Input: part model. Units: mm. Frame: model coordinates. Face numbers are marked on the shaded views. A direction names the side the tool comes from. Round coordinates to 2 decimals unless told otherwise and drop trailing zeros. Write each loop counter-clockwise with the first axis right and the second up, starting at its lowest first coordinate (ties: lowest second). Pieces come first, ordered by that corner, then holes. Notation, with made-up numbers: M 53,-22.75 L 112,-22.75 A12 ccw 112,-8.75 Z; hole C 12.5,34.25 d2. An arc over 180 degrees is marked long. Use one line per item in the form item = value. Start each with the question number.
```python
from build123d import *

# Parameters (mm, degrees)
F0_R      = 25.4
F1_DEPTH  = 31.75
F0_R_2    = 4.7625
F0_R_3    = 6.35
F2_DEPTH  = 12.7
F3_DEPTH  = 6.35
F4_DEPTH  = 25.4
F5_R      = 6.35
F6_DEPTH  = 6.35
F7_DEPTH  = 6.35
F8_R      = 12.7
F10_DEPTH = 31.75
F11_DEPTH = 63.5


with BuildPart() as f1:
    # F0 (on Top) → F1 (new body)
    with BuildSketch(Plane.XY):
        with BuildLine():
            ThreePointArc((19.05, -25.4), (28.3980633142, -14.1990316571), (31.75, 0))
            ThreePointArc((31.75, 0), (28.3980633142, 14.1990316571), (19.05, 25.4))
            ThreePointArc((19.05, 25.4), (14.4949901866, 28.2481461249), (9.525, 30.287569645))
            ThreePointArc((9.525, 30.287569645), (4.8183069939, 31.3822627883), (8.43e-08, 31.75))
            ThreePointArc((8.43e-08, 31.75), (-4.8183069106, 31.3822628011), (-9.525, 30.287569645))
            ThreePointArc((-9.525, 30.287569645), (-14.4949901866, 28.2481461249), (-19.05, 25.4))
            ThreePointArc((-19.05, 25.4), (-26.8271299333, 16.9813898), (-31.1085197333, 6.35))
            ThreePointArc((-31.1085197333, 6.35), (-31.75, 0), (-31.1085197333, -6.35))
            ThreePointArc((-31.1085197333, -6.35), (-26.8271299333, -16.9813898), (-19.05, -25.4))
            ThreePointArc((-19.05, -25.4), (-14.4949901866, -28.2481461249), (-9.525, -30.287569645))
            ThreePointArc((-9.525, -30.287569645), (-4.8183069522, -31.3822627947), (0, -31.75))
            ThreePointArc((0, -31.75), (4.8183069522, -31.3822627947), (9.525, -30.287569645))
            ThreePointArc((9.525, -30.287569645), (14.4949901866, -28.2481461249), (19.05, -25.4))
        make_face()
        Circle(F0_R, mode=Mode.SUBTRACT)
    extrude(amount=F1_DEPTH)

    # F0 (on Top) → F2 (join)
    with BuildSketch(Plane.XY):
        with BuildLine():
            ThreePointArc((9.525, 41.275), (9.2499372193, 43.5475066424), (8.4406353932, 45.6887624719))
            ThreePointArc((8.4406353932, 45.6887624719), (0, 50.8), (-8.4406353932, 45.6887624719))
            ThreePointArc((-8.4406353932, 45.6887624719), (-9.2499372193, 43.5475066424), (-9.525, 41.275))
            ThreePointArc((-9.525, 41.275), (-6.735192061, 34.5398078794), (8.43e-08, 31.75))
            ThreePointArc((8.43e-08, 31.75), (6.7351921206, 34.539807939), (9.525, 41.275))
        make_face()
        with Locations((0, 41.275)):
            Circle(F0_R_2, mode=Mode.SUBTRACT)
        with BuildLine():
            ThreePointArc((8.43e-08, 31.75), (4.8183069939, 31.3822627883), (9.525, 30.287569645))
            Line((9.525, 30.287569645), (9.525, 41.275))
            ThreePointArc((9.525, 41.275), (6.7351921206, 34.539807939), (8.43e-08, 31.75))
        make_face()
        with BuildLine():
            Line((9.525, -41.275), (9.525, -30.287569645))
            ThreePointArc((9.525, -30.287569645), (4.8183069522, -31.3822627947), (0, -31.75))
            ThreePointArc((0, -31.75), (6.7351920908, -34.5398079092), (9.525, -41.275))
        make_face()
        with BuildLine():
            ThreePointArc((-9.525, -41.275), (-6.7351920908, -34.5398079092), (0, -31.75))
            ThreePointArc((0, -31.75), (-4.8183069522, -31.3822627947), (-9.525, -30.287569645))
            Line((-9.525, -30.287569645), (-9.525, -41.275))
        make_face()
        with BuildLine():
            ThreePointArc((-8.4406353932, -45.6887624719), (0, -50.8), (8.4406353932, -45.6887624719))
            ThreePointArc((8.4406353932, -45.6887624719), (9.2499372193, -43.5475066424), (9.525, -41.275))
            ThreePointArc((9.525, -41.275), (6.7351920908, -34.5398079092), (0, -31.75))
            ThreePointArc((0, -31.75), (-6.7351920908, -34.5398079092), (-9.525, -41.275))
            ThreePointArc((-9.525, -41.275), (-9.2499372193, -43.5475066424), (-8.4406353932, -45.6887624719))
        make_face()
        with Locations((0, -41.275)):
            Circle(F0_R_2, mode=Mode.SUBTRACT)
        with BuildLine():
            ThreePointArc((-9.525, 30.287569645), (-4.8183069106, 31.3822628011), (8.43e-08, 31.75))
            ThreePointArc((8.43e-08, 31.75), (-6.735192061, 34.5398078794), (-9.525, 41.275))
            Line((-9.525, 41.275), (-9.525, 30.287569645))
        make_face()
        with BuildLine():
            ThreePointArc((19.05, 25.4), (28.3980633142, 14.1990316571), (31.75, 0))
            ThreePointArc((31.75, 0), (28.3980633142, -14.1990316571), (19.05, -25.4))
            Line((19.05, -25.4), (66.8686259006, -12.245095326))
            ThreePointArc((66.8686259006, -12.245095326), (76.2, 0), (66.8686259006, 12.245095326))
            Line((66.8686259006, 12.245095326), (19.05, 25.4))
        make_face()
        with Locations((63.5, 0)):
            Circle(F0_R_3, mode=Mode.SUBTRACT)
    extrude(amount=F2_DEPTH)

    # F0 (on Top) → F3 (join)
    with BuildSketch(Plane.XY):
        with BuildLine():
            ThreePointArc((-9.525, 41.275), (-9.2499372193, 43.5475066424), (-8.4406353932, 45.6887624719))
            Line((-8.4406353932, 45.6887624719), (-19.05, 25.4))
            ThreePointArc((-19.05, 25.4), (-14.4949901866, 28.2481461249), (-9.525, 30.287569645))
            Line((-9.525, 30.287569645), (-9.525, 41.275))
        make_face()
        with BuildLine():
            ThreePointArc((9.525, 30.287569645), (14.4949901866, 28.2481461249), (19.05, 25.4))
            Line((19.05, 25.4), (8.4406353932, 45.6887624719))
            ThreePointArc((8.4406353932, 45.6887624719), (9.2499372193, 43.5475066424), (9.525, 41.275))
            Line((9.525, 41.275), (9.525, 30.287569645))
        make_face()
        with BuildLine():
            Line((8.4406353932, -45.6887624719), (19.05, -25.4))
            ThreePointArc((19.05, -25.4), (14.4949901866, -28.2481461249), (9.525, -30.287569645))
            Line((9.525, -30.287569645), (9.525, -41.275))
            ThreePointArc((9.525, -41.275), (9.2499372193, -43.5475066424), (8.4406353932, -45.6887624719))
        make_face()
        with BuildLine():
            Line((-19.05, -25.4), (-8.4406353932, -45.6887624719))
            ThreePointArc((-8.4406353932, -45.6887624719), (-9.2499372193, -43.5475066424), (-9.525, -41.275))
            Line((-9.525, -41.275), (-9.525, -30.287569645))
            ThreePointArc((-9.525, -30.287569645), (-14.4949901866, -28.2481461249), (-19.05, -25.4))
        make_face()
    extrude(amount=F3_DEPTH)

    # F0 (on Top) → F4 (join)
    with BuildSketch(Plane.XY):
        with BuildLine():
            ThreePointArc((-31.1085197333, -6.35), (-31.75, 0), (-31.1085197333, 6.35))
            Line((-31.1085197333, 6.35), (-57.15, 6.35))
            Line((-57.15, 6.35), (-57.15, 0))
            Line((-57.15, 0), (-57.15, -6.35))
            Line((-57.15, -6.35), (-31.1085197333, -6.35))
        make_face()
    extrude(amount=F4_DEPTH)

    # F5 (on Front) → F6 (cut, symmetric)
    with BuildSketch(Plane.XZ):
        with Locations((-44.4733425975, 12.6999998465)):
            Circle(F5_R)
    extrude(amount=F6_DEPTH, both=True, mode=Mode.SUBTRACT)

    # F5 (on Front) → F7 (cut, symmetric)
    with BuildSketch(Plane.XZ):
        with Locations((-44.4733425975, 12.6999998465)):
            Circle(F5_R)
    extrude(amount=F7_DEPTH, both=True, mode=Mode.SUBTRACT)

    # F8
    f8_edges = [f1.edges().sort_by_distance(p)[0] for p in [
        (-57.15, 0, 25.4),
    ]]
    fillet(f8_edges, radius=F8_R)

    # F9 (on Right) → F10 (cut)
    with BuildSketch(Plane.YZ):
        Polygon((0, 31.75), (-7.9375, 31.75), (-7.9375, 12.7), (7.9375, 12.7), (7.9375, 31.75), align=None)
    extrude(amount=F10_DEPTH, mode=Mode.SUBTRACT)

    # F9 (on Right) → F11 (cut)
    with BuildSketch(Plane.YZ):
        Polygon((0, 31.75), (-7.9375, 31.75), (-7.9375, 12.7), (7.9375, 12.7), (7.9375, 31.75), align=None)
    extrude(amount=F11_DEPTH, mode=Mode.SUBTRACT)


solid = f1.part
```
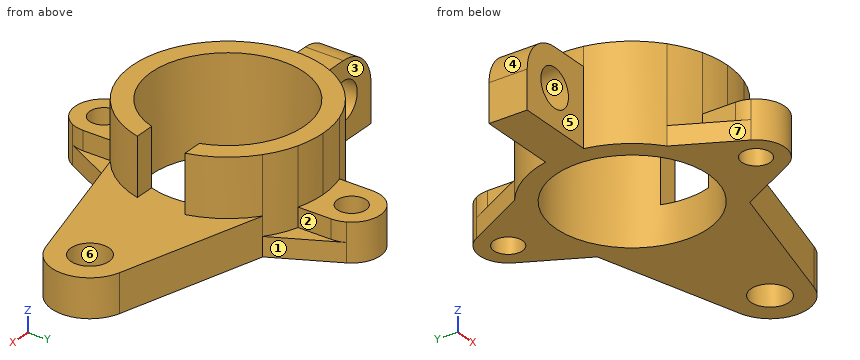
Item 1: Cut plane A-A (y = 0). Output: boundary loops of the cut face in (x, z), plus the area to 3 significant figures.
Item 2: First-contact query: pin 1 (5.5 mm diameter, centred on x = 0, y = -41.275, fed in from +Z); pin 2 (1.9 mm diameter, centred on y = -35, z = 10, fed in from -X) (3 decimals); pin 3 (1 mm diameter, centred on y = -3.5, z = 4, fed in from +X); pin 4 (10 mm diameter, centred on x = -37.5, y = -1.5, fed in from +Z). Flat tips, straight axial feed; report the tip coordinate or a pass-through.
Item 3: Ray query, line 1 (Y direction, x = 0, z = 9.25); line 2 (X direction, y = 0, z = 13); line 3 (Y direction, x = -2.5, z = 9). Return the intervals inside material, ascending. Write a range as from..to.
Item 4: Cut plane D-D (y = -21.5). Output: boundary loops of the cut face in (x, z).
Item 5: Reachability of the marked faces 1, 2, 3, 4 and 5 from +Z, -Z, +X, -X, +Y, -Y: full face, straight path, thin tool, end or side. Return the list, or none.
Item 6: Draft query along Y for the marked faces 6, 7 and 8. Return one class per face: +Y half, -Y half, draft (parallel to the pull), parting line (faces both ways), or undercut.
Item 7: Cut plane B-B (z = 3). Give the number of separate pieces and of enclosed holes in the cut face, plus the area to 3 significant figures.
Item 8: Cut plane C-C (x = 64.5). Output: boundary loops of the cut face in (y, z), plus the area to 3 significant figures.
Final values:
q1.outline = M -57.15,0 L -25.4,0 L -25.4,31.75 L -31.75,31.75 L -31.75,25.4 L -44.45,25.4 A12.7 ccw -57.15,12.7 Z; M 25.4,0 L 57.15,0 L 57.15,12.7 L 25.4,12.7 Z; M 69.85,0 L 76.2,0 L 76.2,12.7 L 69.85,12.7 Z; hole C -44.47,12.7 d12.7
q1.area = 1,170 mm^2
q2.pin_1 = through
q2.pin_2 = -9.525
q2.pin_3 = 75.84
q2.pin_4 = 25.4
q3.line_1 = -50.8..-46.04, -36.51..-25.4, 25.4..36.51, 46.04..50.8
q3.line_2 = -57.15..-50.82, -38.13..-25.4
q3.line_3 = -50.47..-45.33, -37.22..-25.28, 25.28..37.22, 45.33..50.47
q4.outline = M -23.36,0 L -13.52,0 L -13.52,31.75 L -23.36,31.75 Z; M 13.52,0 L 33.23,0 L 33.23,12.7 L 23.36,12.7 L 23.36,31.75 L 13.52,31.75 Z
q5.face_1 = +Z, -Z, +X, +Y
q5.face_2 = +Z, +X, +Y
q5.face_3 = +Z, -Z, -X, +Y
q5.face_4 = +Z, -X, +Y, -Y
q5.face_5 = +Z, -Z, -X, -Y
q6.face_6 = undercut
q6.face_7 = -Y half
q6.face_8 = draft
q7.separate_pieces = 1
q7.enclosed_holes = 4
q7.area = 3,620 mm^2
q8.outline = M -12.9,0 L -6.27,0 L -6.27,12.7 L -12.9,12.7 Z; M 6.27,0 L 12.9,0 L 12.9,12.7 L 6.27,12.7 Z
q8.area = 168 mm^2
